```python
from build123d import *

# Parameters (mm, degrees)
F0_W     = 60.96
F0_H     = 60.96
F0_R     = 6.35
F1_DEPTH = 2.54
F2_DEPTH = 50.8
F0_H_2   = 1.27
F3_DEPTH = 48.26


with BuildPart() as f1:
    # F0 (on Top) → F1 (new body)
    with BuildSketch(Plane.XY):
        Rectangle(F0_W, F0_H)
        Circle(F0_R, mode=Mode.SUBTRACT)
    extrude(amount=F1_DEPTH)

    # F0 (on Top) → F2 (join)
    with BuildSketch(Plane.XY):
        Polygon((-30.48, -30.48), (-30.48, 30.48), (-30.48, 31.75), (-31.75, 31.75), (-31.75, -31.75), (-30.48, -31.75), align=None)
        Polygon((30.48, 31.75), (30.48, 30.48), (30.48, -30.48), (30.48, -31.75), (31.75, -31.75), (31.75, 31.75), align=None)
    extrude(amount=F2_DEPTH)

    # F0 (on Top) → F3 (join)
    with BuildSketch(Plane.XY):
        with Locations((0, -31.115)):
            Rectangle(F0_W, F0_H_2)
        with Locations((0, 31.115)):
            Rectangle(F0_W, F0_H_2)
    extrude(amount=F3_DEPTH)


solid = f1.part
```
Geometry: final body of the model. Coordinates: model frame, mm. A direction names the side the tool comes from. Coordinates: 2 decimals unless noted, no trailing zeros. Order: outer loops, then holes, each group sorted by start corner. A loop starts at its lowest first (then second) coordinate and runs counter-clockwise, first axis right, second up. Notation, with made-up numbers: (63, 11) - (85, 11) arc R24 cw to (85, 35) - close; hole circle Ø6 at (-37, -37). An arc over 180 degrees is marked (long way). Return JSON: item names as keys, results as strings. Group by question number.
1. Material intervals for line 1 along Y through (x, z) = (-29, 18.5); line 2 along Y through (x, z) = (0, 1.1), sorted ascending. Write a range as [from, to].
2. Cut plane D-D (y = 18). Output: boundary loops of the cut face in (x, z).
3. Pull-direction query (X, two-part tool) for faces 3 (the face through (7, 0, 0)), 4 (the face through (-31.75, 0, 25)), 5 (the face through (30.48, 0, 26)); classes: pulls with the +X half, pulls with the -X half, needs draft (parallel to the pull), parting line crosses it, or undercut.
4. Cut plane C-C (y = 0). Output: boundary loops of the cut face in (x, z).
5. Set-up query: faces 1 (the face through (-1.38, -6.2, 1.25)), 2 (the face through (0, 30.48, 25)). Return all of +Z, -Z, +X, -X, +Y, -Y with unobstructed straight access to the full face (end or side cutting, diameter ignored); none if empty.
6. Cut plane A-A (x = 0). Output: boundary loops of the cut face in (y, z).
7. Cut plane B-B (z = 24). Output: boundary loops of the cut face in (x, y), plus the area to 3 significant figures.
8. Pin query (flat end, axial travel): pin 1 (8 mm diameter, centred on x = 0, y = 14.5, fed in from +Z); pin 2 (1 mm diameter, centred on x = 18, y = -22, fed in from -Z); pin 3 (1.4 mm diameter, centred on x = 13.5, y = 31.5, fed in from +Z); pin 4 (10 mm diameter, centred on x = 0, y = 0, fed in from +Z). Return the tip coordinate at first contact, or that it passes through.
Resolved:
{
 "1": {"line 1": "y = [-31.75, -30.48], [30.48, 31.75]", "line 2": "y = [-31.75, -6.35], [6.35, 31.75]"},
 "2": {"outline": "(-31.75, 0) - (31.75, 0) - (31.75, 50.8) - (30.48, 50.8) - (30.48, 2.54) - (-30.48, 2.54) - (-30.48, 50.8) - (-31.75, 50.8) - close"},
 "3": {"face 3": "needs draft", "face 4": "pulls with the -X half", "face 5": "undercut"},
 "4": {"outline": "(-31.75, 0) - (-6.35, 0) - (-6.35, 2.54) - (-30.48, 2.54) - (-30.48, 50.8) - (-31.75, 50.8) - close; (6.35, 0) - (31.75, 0) - (31.75, 50.8) - (30.48, 50.8) - (30.48, 2.54) - (6.35, 2.54) - close"},
 "5": {"face 1": "+Z, -Z", "face 2": "+Z"},
 "6": {"outline": "(-31.75, 0) - (-6.35, 0) - (-6.35, 2.54) - (-30.48, 2.54) - (-30.48, 48.26) - (-31.75, 48.26) - close; (6.35, 0) - (31.75, 0) - (31.75, 48.26) - (30.48, 48.26) - (30.48, 2.54) - (6.35, 2.54) - close"},
 "7": {"outline": "(-31.75, -31.75) - (31.75, -31.75) - (31.75, 31.75) - (-31.75, 31.75) - close; hole (-30.48, -30.48) - (30.48, -30.48) - (30.48, 30.48) - (-30.48, 30.48) - close", "area": "316 mm²"},
 "8": {"pin 1": "stops at z = 2.54", "pin 2": "stops at z = 0", "pin 3": "stops at z = 48.26", "pin 4": "passes through"}
}
